Can you work these out from the model? Positions are in its coordinate system, mm. A direction names the side the tool comes from. Give positions to 0.01 mm unless a question says otherwise; leave off trailing zeros. Order: outer loops, then holes, each group sorted by start corner. A loop starts at its lowest first (then second) coordinate and runs counter-clockwise, first axis right, second up. Notation, with made-up numbers: M -34,-19 L 0,-19 A9 cw 0,-10 Z; hole C 57.25,-34 d10. An arc over 180 degrees is marked long. Write each question's results on one line, items separated by ' | '.
Autodesk Inventor part; units mm, degrees
ref_plane "YZ Plane" through (0, 0, 0) normal (1, 0, 0) x (0, 1, 0)
ref_plane "XZ Plane" through (0, 0, 0) normal (0, 1, 0) x (-1, 0, 0)
ref_plane "XY Plane" through (0, 0, 0) normal (0, 0, 1) x (1, 0, 0)
sketch "Sketch1" plane through (0, 0, 0) normal (0, 0, 1) x (1, 0, 0)
  line L0 (0, 0) -> (12.7, 0)
  line L1 (12.7, 0) -> (12.7, 3.175)
  line L2 (12.7, 3.175) -> (0, 3.175)
  line L3 (0, 3.175) -> (0, 0)
  line L4 (-3.6576, 41.275) -> (16.3322, 41.275)
  line L5 (16.3322, 41.275) -> (16.3322, 3.175)
  line L6 (16.3322, 3.175) -> (-3.6576, 3.175)
  line L7 (-3.6576, 3.175) -> (-3.6576, 41.275)
  point P0 (16.3322, 22.225)
  point P1 (-3.6576, 22.225)
  point P2 (12.7, 3.175)
  point P3 (0, 3.175)
  dimension "d0" = 12.7
  dimension "d1" = 3.175
  dimension "d2" = 19.9898
  dimension "d3" = 3.6576
  dimension "d4" = 38.1
extrude "Extrusion1" add sketch "Sketch1" along normal blind 3.175
properties part number "servo short side"
(1) Will these pins go through, and if not, where does the flat tip stop? P1, Ø1.6, axis at y = 1.5, z = 1.5, coming from the -X side; P2, Ø1.6, axis at y = 1.5, z = 1.5, coming from the +X side; P3, Ø1, axis at x = -1, z = 2.5, coming from the -Y side (3 decimals).
Data:
P1: stops at x = 0 | P2: stops at x = 12.7 | P3: stops at y = 3.175
(2) For faces 1 (the face through (-2, 3.175, 2)), 2 (the face through (-3.658, 22, 2)), 3 (the face through (12.7, 2, 2)), which set-ups out of +Z, -Z, +X, -X, +Y, -Y let a thin tool reach every point of the face, with its end or its side?
Data:
face 1: +Z, -Z, -X, -Y | face 2: +Z, -Z, -X, +Y, -Y | face 3: +Z, -Z, +X, -Y
(3) Imagine slicing it at B-B, the plane x = -2.25. Write out the boundary of the cut face in (y, z) (3 decimals).
Data:
outline: M 3.175,0 L 41.275,0 L 41.275,3.175 L 3.175,3.175 Z
(4) Imagine slicing it at A-A, the plane z = 2.1. Write out the boundary of the cut face in (x, y) (3 decimals), plus the area to 3 significant figures.
Data:
outline: M -3.658,3.175 L 0,3.175 L 0,0 L 12.7,0 L 12.7,3.175 L 16.332,3.175 L 16.332,41.275 L -3.658,41.275 Z | area: 802 mm2
(5) I need wall thicknesses on L1, parallel to Y at x = 14.75, z = 2.2 (3 decimals); L2, parallel to X at y = 3, z = 0.45. Which ranges of each line are inside material? Lowest first, please. Write a range as from..to.
Data:
L1: y = 3.175..41.275 | L2: x = 0..12.7
